Autodesk Fusion 360 part; units mm, degrees
sketch "Sketch1" plane through (0, 0, 0) normal (0, 1, 0) x (1, 0, 0)
  line L0 (-40, 35) -> (31, 35)
  line L1 (31, 35) -> (31, -20)
  line L2 (31, -20) -> (-40, -20)
  line L3 (-40, -20) -> (-40, 35)
  line L4 (-40, 35) -> (-45, 35)
  line L5 (-45, 35) -> (-45, -20)
  line L6 (-45, -20) -> (-40, -20)
  line L7 (-40, -20) -> (-40, 35)
  dimension "d1" = 71
  dimension "d2" = 55
extrude "Extrude1" add sketch "Sketch1" along normal blind 3 contours L0 L1 L2 L3 L7 makes body 1
extrude "Extrude2" add sketch "Sketch1" along normal blind 3 contours L3 L4 L5 L6 L7 bodies 1
extrude "Extrude3" add sketch "Sketch1" along normal blind 29 separate body contours L3 L4 L5 L6 L7 makes body 2
sketch "Sketch2" plane through (-40, 0, 0) normal (1, 0, 0) x (0, 0, -1)
  line L0 (-20, 0) -> (35, 0)
  line L1 (35, 0) -> (35, 29)
  line L2 (35, 29) -> (-20, 29)
  line L3 (-20, 29) -> (-20, 0)
  line L4 (35, 29) -> (-1, 29)
  line L5 (-1, 29) -> (-1, 3)
  line L6 (-1, 3) -> (35, 3)
  line L7 (35, 3) -> (35, 29)
  line L8 (-20, 3) -> (35, 3)
  dimension "d9" = 36
extrude "Extrude4" add sketch "Sketch2" along normal blind 4 contours L1 L2 L4 L5 L6 L7 L8 bodies 1 2
sketch "Sketch3" plane through (-36, 0, 0) normal (1, 0, 0) x (0, 0, -1)
  line L0 (-1, 29) -> (-1, 3)
  line L1 (-1, 3) -> (35, 3)
  line L2 (35, 3) -> (35, 29)
  line L3 (35, 29) -> (-1, 29)
  line L4 (20.1451, 29) -> (20.1451, 23.5)
  line L5 (-1, 23.5) -> (24, 23.5)
  line L6 (24, 23.5) -> (24, 8.5)
  line L7 (24, 8.5) -> (-1, 8.5)
  line L8 (-1, 8.5) -> (-1, 23.5)
  dimension "d12" = 5.5
  dimension "d13" = 25
  dimension "d14" = 15
extrude "Extrude5" add sketch "Sketch3" along normal blind 3 contours L0 L5 L6 L7 L8 bodies 1
fillet "Fillet1" radius 2 4 edges at (-34.5, 23.5, 1) (-34.5, 8.5, 1) (-34.5, 23.5, -24) (-34.5, 8.5, -24) on bodies 1
sketch "Sketch4" plane through (-40, 0, 0) normal (1, 0, 0) x (0, 0, -1)
  line L0 (-20, 3) -> (-1, 3)
  line L1 (-1, 3) -> (-1, 29)
  line L2 (-1, 29) -> (-20, 29)
  line L3 (-20, 29) -> (-20, 3)
  line L4 (-11.8235, 29) -> (-11.8235, 22.5)
  line L5 (-20, 22.5122) -> (-10.75, 22.5122)
  dimension "d18" = 6.5
  dimension "d19" = 9.25
sketch "Sketch5" plane through (-45, 0, 0) normal (-1, 0, 0) x (0, 0, 1)
  line L0 (-35, 0) -> (20, 0)
  line L1 (20, 0) -> (20, 29)
  line L2 (20, 29) -> (-35, 29)
  line L3 (-35, 29) -> (-35, 0)
  line L4 (8.25, 22.5122) -> (8.25, 13.0122)
  line L5 (8.25, 13.0122) -> (10.25, 13.0122)
  dimension "d22" = 9.5
  dimension "d23" = 2
cylinder "CylinderPrimitive2" add diameter 4 height 6 placed x (0, 0, -1) y (0, 1, 0) z (1, 0, 0) at (-40, 13.0122, 10.25) bodies 1
extrude "Extrude6" add 1 faces at (8.6667, 3, -4.6667) along direction (0, 1, 0) blind 2 on bodies 1 bodies 1
extrude "Extrude7" cut 1 faces at (5.6667, 0, 1.6667) along direction (0, 1, 0) blind 2 on bodies 1 bodies 1
cylinder "CylinderPrimitive3" cut diameter 6 height -6 placed x (0, 0, -1) y (0, 1, 0) z (1, 0, 0) at (-40, 22.5122, 10.75) bodies 1
extrude "Extrude8" add 1 faces at (5.6667, 2, 1.6667) along direction (0, -1, 0) blind 2 on bodies 1 bodies 1
sketch "Sketch8" plane through (0, 0, 0) normal (0, -1, 0) x (1, 0, 0)
  line L0 (-45, -35) -> (31, -35)
  line L1 (31, -35) -> (31, 20)
  line L2 (31, 20) -> (-45, 20)
  line L3 (-45, 20) -> (-45, -35)
  line L4 (31, 20) -> (6, 20)
  line L5 (6, 20) -> (1, 20)
  line L6 (1, 20) -> (1, -35)
  line L7 (1, -35) -> (6, -35)
  line L8 (6, -35) -> (6, 20)
  dimension "d34" = 25
  dimension "d35" = 5
extrude "Extrude9" cut sketch "Sketch8" against normal blind 2 contours L0 L2 L5 L6 L7 L8 bodies 1
chamfer "Chamfer1" distance 2 angle 45 2 edges at (3.5, 2, 20) (3.5, 2, -35) on bodies 1
extrude "Extrude10" cut 1 faces at (31, 3.3333, -16.6667) along direction (-1, 0, 0) blind 10 on bodies 1 bodies 1
sketch "Sketch9" plane through (-45, 0, 0) normal (-1, 0, 0) x (0, 0, 1)
  circle A0 centre (10.75, 22.5122) radius 3
  line L0 (20, 0) -> (20, 29)
  line L1 (20, 29) -> (-35, 29)
  line L2 (-35, 29) -> (-35, 0)
  line L3 (-35, 0) -> (20, 0)
  line L4 (-20, 29) -> (-15, 29)
  line L5 (-15, 29) -> (-20, 29)
  line L6 (-20, 29) -> (-20, 0)
  line L7 (-20, 0) -> (-15, 0)
  line L8 (-15, 0) -> (-15, 29)
  dimension "d41" = 20
extrude "Extrude11" cut sketch "Sketch9" against normal blind 1 contours L1 L3 L4 L5 L6 L7 L8 bodies 1
chamfer "Chamfer2" distance 2 angle 45 2 edges at (-44, 29, -17.5) (-44, 0, -17.5) on bodies 1
Verification items for the finished model (mm, model axes). A direction names the side the tool comes from. Coordinates: 2 decimals unless noted, no trailing zeros. Order: outer loops, then holes, each group sorted by start corner. A loop starts at its lowest first (then second) coordinate and runs counter-clockwise, first axis right, second up. Notation, with made-up numbers: (52.5, 47) -> (83.5, 47) arc R22 ccw to (83.5, 70) -> close; hole circle Ø2 at (31, -8.5). An arc over 180 degrees is marked (long way). Use CSV: the item, a comma, the result in double quotes. Start each with the question number.
Q1. Tool access check on faces 1 (the flat face through (-43, 28, -17)), 2 (the flat face through (-43, 1, -17)), 3 (the flat face through (-37, 17, 1)). Record the directions out of +Z, -Z, +X, -X, +Y, -Y that give a thin tool (end or side, any length) a straight path to the whole face; none if there is none.
Q2. Draft check along Y on faces 4 (the cylindrical face through (-34.48, 9.07, -23.4)), 5 (the flat face through (-45, 15, -28)), 6 (the cylindrical face through (-42.46, 24.54, 12.96)), 7 (the flat face through (4, 3, -34)). Enter one of: +Y half, -Y half, draft (parallel to the pull), parting line (faces both ways), or undercut.
Q3. Depth check by flat-ended pin: P1, Ø3, axis at y = 9, z = -1.5, coming from the +X side; P2, Ø3.5, axis at x = -34, y = 16, coming from the -Z side; P3, Ø3.5, axis at x = -34, z = -7.5, coming from the +Y side. Enter the tip coordinate at first touch or a pass-through.
Q4. Section check B-B, the plane z = -27. Record the cut outline in (x, y).
Q5. Section check D-D, the plane z = -5. Record the cut outline in (x, y).
Q6. Section check C-C, the plane x = -31. Record the cut outline in (y, z), and give its area (3 significant figures).
Q7. Section check A-A, the plane z = 10.25. Record the cut outline in (x, y), and give its area (3 significant figures).
Q8. Thickness scan on line 1 along Y through (x, z) = (-41.85, 10.75); line 2 along Y through (x, z) = (4, 10); line 3 along X through (y, z) = (18, 6). Record the ranges inside material, lowest first.
Returned:
1,face 1,"-X, +Y"
1,face 2,"-X, -Y"
1,face 3,"+X, +Y"
2,face 4,"undercut"
2,face 5,"draft"
2,face 6,"undercut"
2,face 7,"-Y half"
3,P1,"stops at x = -33"
3,P2,"stops at z = -24"
3,P3,"stops at y = 23.5"
4,outline,"(-45, 0) -> (1, 0) -> (1, 2) -> (6, 2) -> (6, 0) -> (21, 0) -> (21, 5) -> (-36, 5) -> (-36, 29) -> (-45, 29) -> close"
5,outline,"(-45, 0) -> (1, 0) -> (1, 2) -> (6, 2) -> (6, 0) -> (21, 0) -> (21, 5) -> (-36, 5) -> (-36, 8.5) -> (-33, 8.5) -> (-33, 23.5) -> (-36, 23.5) -> (-36, 29) -> (-45, 29) -> close"
6,outline,"(0, -35) -> (5, -35) -> (5, 20) -> (0, 20) -> close"
6,area,"275 mm^2"
7,outline,"(-45, 0) -> (1, 0) -> (1, 2) -> (6, 2) -> (6, 0) -> (21, 0) -> (21, 5) -> (-40, 5) -> (-40, 11.01) -> (-34, 11.01) -> (-34, 15.01) -> (-40, 15.01) -> (-40, 19.55) -> (-45, 19.55) -> close; (-45, 25.47) -> (-40, 25.47) -> (-40, 29) -> (-45, 29) -> close"
7,area,"434 mm^2"
8,line 1,"y = 0 to 19.51, 25.51 to 29"
8,line 2,"y = 2 to 5"
8,line 3,"x = -45 to -40"
